```python
from build123d import *

# Parameters (mm, degrees)
F1_DEPTH = 10
F2_COUNT = 8
F3_R     = 0.4


with BuildPart() as f1:
    # F0 (on Top) → F1 (new body)
    with BuildSketch(Plane.XY):
        with BuildLine():
            add(Edge.make_bspline(
                [(-14.9177111461, 20.0614529425), (-23.5650084882, 44.8479673469), (-2.5884105388, 70.4783619432), (0, 85)],
                knots=[18.3724715396, 18.3724715396, 18.3724715396, 18.3724715396, 85, 85, 85, 85], degree=3))
            ThreePointArc((-14.9177111461, 20.0614529425), (-7.8569611313, 23.7332711985), (0, 25))
            Line((0, 25), (0, 85))
        make_face()
        with BuildLine():
            ThreePointArc((0, 25), (7.8569611313, 23.7332711985), (14.9177111461, 20.0614529425))
            add(Edge.make_bspline(
                [(14.9177111461, 20.0614529425), (23.5650084882, 44.8479673469), (2.5884105388, 70.4783619432), (0, 85)],
                knots=[18.3724715396, 18.3724715396, 18.3724715396, 18.3724715396, 85, 85, 85, 85], degree=3))
            Line((0, 85), (0, 25))
        make_face()
        with BuildLine():
            add(Edge.make_bspline(
                [(0, 0), (7.8962181087, 6.4559084388), (12.5332279154, 13.2265974258), (14.9177111461, 20.0614529425)],
                knots=[0, 0, 0, 0, 18.3724715396, 18.3724715396, 18.3724715396, 18.3724715396], degree=3))
            ThreePointArc((14.9177111461, 20.0614529425), (7.8569611313, 23.7332711985), (0, 25))
            ThreePointArc((0, 25), (-7.8569611313, 23.7332711985), (-14.9177111461, 20.0614529425))
            add(Edge.make_bspline(
                [(0, 0), (-7.8962181087, 6.4559084388), (-12.5332279154, 13.2265974258), (-14.9177111461, 20.0614529425)],
                knots=[0, 0, 0, 0, 18.3724715396, 18.3724715396, 18.3724715396, 18.3724715396], degree=3))
        make_face()
    extrude(amount=F1_DEPTH)

    # F2: F1 ×8 about axis
    f2_axis = Axis((0, 0, 5), (0, 0, -1))


with BuildPart() as f1_1:
    add(f1.part)
    for i in range(1, F2_COUNT):
        add(f1.part.rotate(f2_axis, i * 360 / F2_COUNT))

    # F3
    f3_edges = [f1_1.edges().sort_by_distance(p)[0] for p in [
        (60.104076, 60.104076, 5),
        (85, 0, 5),
        (60.104076, -60.104076, 5),
        (0, -85, 5),
        (0, 85, 5),
        (-60.104076, 60.104076, 5),
        (-85, 0, 5),
        (-60.104076, -60.104076, 5),
    ]]
    fillet(f3_edges, radius=F3_R)


solid = f1_1.part
```
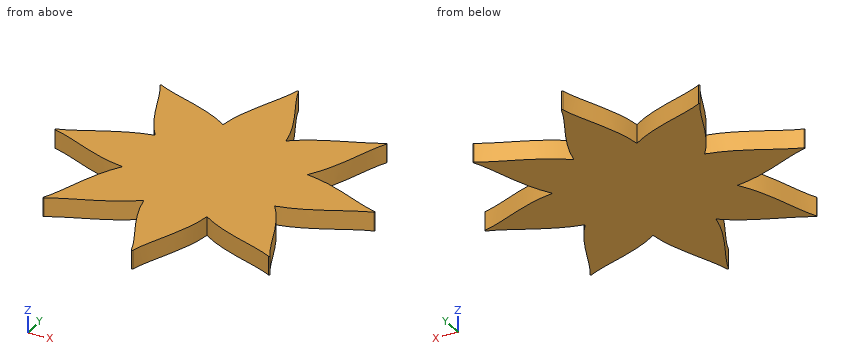
Input: part model. Units: mm. Frame: model coordinates. Give positions to 0.01 mm unless a question says otherwise; leave off trailing zeros. Write item = value, one per line. Start each with the question number.
1. Section query A-A, the plane x = 45. Count the separate pieces of the cut face and the enclosed holes in it, then the cut area to 3 significant figures.
2. First-contact query: pin 1 Ø5 at (x, z) = (-11.5, 2) entering from +Y; pin 2 Ø1.5 at (x, z) = (-33, 8.5) entering from -Y; pin 3 Ø2 at (y, z) = (40, 3.5) entering from -X. Flat tips, straight axial feed; report the tip coordinate or a pass-through.
3. Ray query, L1, parallel to Y at x = 44, z = 1.75; L2, parallel to Y at x = -42, z = 7.25; L3, parallel to X at y = 45.5, z = 2.5 (3 decimals). Return the intervals inside material, ascending.
Check sheet entries:
q1.separate_pieces = 3
q1.enclosed_holes = 0
q1.area = 874 mm2
q2.pin_1 = 62.69
q2.pin_2 = -49.02
q2.pin_3 = -51.84
q3.L1 = -52.94 to -23.17, -15.63 to 15.63, 23.17 to 52.94
q3.L2 = -52.21 to -19.8, -16.05 to 16.05, 19.8 to 52.21
q3.L3 = -53.495 to -25.995, -15.268 to 15.268, 25.995 to 53.495
